Design review of the part built by this model. Coordinates are the model's own, in mm. A direction names the side the tool comes from. Coordinates: 2 decimals unless noted, no trailing zeros. Loops run counter-clockwise (first coordinate to the right, second up) from the corner with the lowest first, then second, coordinate; pieces in that order, holes last. Notation, with made-up numbers: M 14,-25 L 19,-25 A34 cw 19,10 Z; hole C 48,78.5 d10. An arc over 180 degrees is marked long. Put each result on its own line as item: value. Start each with the question number.
(1) The part is to be moulded in two halves that separate along Z. For faces 5 (the flat face through (8.71, -17.16, -3.14)), 6 (the cylindrical face through (13.768, 14.235, -2.872)), say which applies: +Z half, -Z half, draft (parallel to the pull), parting line (faces both ways), or undercut.
(2) For probe 1 along Z at (x, y) = (7.7, -12.5); probe 2 along Y at (x, z) = (14.25, -3.1); probe 3 along Y at (x, z) = (4.25, -3.25), list the stretches that pass through material, from the lowest coordinate up. Write a range as [from, to].
(3) Take a section at A-A, the plane z = -7. Give the boundary of the cut face in (x, y).
(4) Take a section at D-D, the plane x = 13.5. Give the boundary of the cut face in (y, z).
(5) Take a section at B-B, the plane x = 9. Give the boundary of the cut face in (y, z), then the cut area to 3 significant figures.
(6) Clearance check with a flat-ended pin moving along its axis: pin 1 (0.5 mm diameter, centred on y = 12.5, z = -4, fed in from +X). State where the tip first meets the part, or that it passes through.
(7) Take a section at C-C, the plane y = -6. Give the boundary of the cut face in (x, z).
(8) For faces 1 (the flat face through (8.71, 17.16, -3.14)), 2 (the flat face through (10.8, 24, -3)), 3 (the flat face through (10.8, -24, -3)), 4 (the flat face through (9.8, 12, -5)), list the 3-axis set-ups (+Z, -Z, +X, -X, +Y, -Y) from which the entire face can be reached by the end or side of a thin tool; tool diameter is ignored.
```python
from build123d import *

# Parameters (mm, degrees)
ESQUISSE1_W                           = 15
ESQUISSE1_H                           = 10
BOSS_EXTRU_1_DEPTH                    = 25
ENL_VEMENT_START                      = -6.2
ENL_VEMENT_DE_MATI_RE_BALAYAGE1_DEPTH = 6.2
ENL_V_MAT_EXTRU_1_REACH               = 32.822
ESQUISSE4_R                           = 1.75
ENL_V_MAT_EXTRU_2_REACH               = 32.822
ESQUISSE5_W                           = 2.7
ESQUISSE5_H                           = 5.9


# Read off the part's stored shape, not the designer's step: Enlèvement de matière-Balayage1
with BuildPart() as part:
    # Esquisse1 → Boss.-Extru.1 (new body)
    with BuildSketch(Plane(origin=(0, 0, 0), x_dir=(1, 0, 0), z_dir=(0, 1, 0))):
        with Locations((7.5, 5)):
            Rectangle(ESQUISSE1_W, ESQUISSE1_H)
    extrude(amount=BOSS_EXTRU_1_DEPTH)

    # Enlèvement de matière-Balayage1 outline → Enlèvement de matière-Balayage1 (cut)
    with BuildSketch(Plane.XY.offset(ENL_VEMENT_START)):
        with BuildLine():
            Line((10.8, 25), (10.8, 22.058471581))
            ThreePointArc((10.8, 22.058471581), (10.4896694, 20.777243155), (9.627466942, 19.780017862))
            Line((9.627466942, 19.780017862), (5.977561393, 17.172942469))
            ThreePointArc((5.977561393, 17.172942469), (4.376328258, 15.320952639), (3.8, 12.941528419))
            Line((3.8, 12.941528419), (3.8, 12.264761516))
            ThreePointArc((3.8, 12.264761516), (4.474960485, 9.702727678), (6.324622072, 7.805798302))
            Line((6.324622072, 7.805798302), (15, 2.600571545))
            Line((15, 2.600571545), (15, 4.466476152))
            Line((15, 4.466476152), (7.14781528, 9.177786983))
            ThreePointArc((7.14781528, 9.177786983), (5.867280336, 10.491045782), (5.4, 12.264761516))
            Line((5.4, 12.264761516), (5.4, 12.941528419))
            ThreePointArc((5.4, 12.941528419), (5.798996486, 14.58882211), (6.907542503, 15.870968915))
            Line((6.907542503, 15.870968915), (10.557448052, 18.478044308))
            ThreePointArc((10.557448052, 18.478044308), (11.912337628, 20.045112625), (12.4, 22.058471581))
            Line((12.4, 22.058471581), (12.4, 25))
            Line((12.4, 25), (10.8, 25))
        make_face()
    extrude(amount=ENL_VEMENT_DE_MATI_RE_BALAYAGE1_DEPTH, mode=Mode.SUBTRACT)

    # Esquisse4 → Enlèv. mat.-Extru.1 (cut, up to next)
    with BuildSketch(Plane(origin=(15, 0, 0), x_dir=(0, 0, -1), z_dir=(1, 0, 0)), mode=Mode.PRIVATE) as enl_v_mat_extru_1_sk1:
        with Locations((3.1, 12.5)):
            Circle(ESQUISSE4_R)
    enl_v_mat_extru_1_tool1 = extrude(enl_v_mat_extru_1_sk1.sketch, amount=-ENL_V_MAT_EXTRU_1_REACH, mode=Mode.PRIVATE) & part.part
    add(enl_v_mat_extru_1_tool1.solids().sort_by_distance((15, 12.5, -3.1))[0], mode=Mode.SUBTRACT)

    # Esquisse5 → Enlèv. mat.-Extru.2 (cut, up to next)
    with BuildSketch(Plane.XY, mode=Mode.PRIVATE) as enl_v_mat_extru_2_sk1:
        with Locations((11.15, 12.5)):
            Rectangle(ESQUISSE5_W, ESQUISSE5_H)
    enl_v_mat_extru_2_tool1 = extrude(enl_v_mat_extru_2_sk1.sketch, amount=-ENL_V_MAT_EXTRU_2_REACH, mode=Mode.PRIVATE) & part.part
    add(enl_v_mat_extru_2_tool1.solids().sort_by_distance((11.15, 12.5, 0))[0], mode=Mode.SUBTRACT)

    # Symétrie1: part across plane


with BuildPart() as part_1:
    add(part.part)
    add(part.part.mirror(Plane(origin=(0, 0, 0), x_dir=(0, 0, 1), z_dir=(0, -1, 0))))


solid = part_1.part
```
Computed values:
1. face 5: draft
1. face 6: undercut
2. probe 1: z = [-10, -4.85], [-1.35, 0]
2. probe 2: y = [-25, -14.25], [-10.75, -4.92], [-3.05, 3.05], [4.92, 10.75], [14.25, 25]
2. probe 3: y = [-25, -15.06], [-10.15, 10.15], [15.06, 25]
3. outline: M 0,-25 L 15,-25 L 15,25 L 0,25 Z; hole M 9.8,-15.45 L 12.5,-15.45 L 12.5,-9.55 L 9.8,-9.55 Z; hole M 9.8,9.55 L 12.5,9.55 L 12.5,15.45 L 9.8,15.45 Z
4. outline: M -25,-10 L 25,-10 L 25,0 L 5.37,0 L 5.37,-6.2 L 3.5,-6.2 L 3.5,0 L -3.5,0 L -3.5,-6.2 L -5.37,-6.2 L -5.37,0 L -25,0 Z; hole C -12.5,-3.1 d3.5; hole C 12.5,-3.1 d3.5
5. outline: M -25,-10 L 25,-10 L 25,0 L 19.33,0 L 19.33,-6.2 L 17.37,-6.2 L 17.37,0 L 8.07,0 L 8.07,-6.2 L 6.2,-6.2 L 6.2,0 L -6.2,0 L -6.2,-6.2 L -8.07,-6.2 L -8.07,0 L -17.37,0 L -17.37,-6.2 L -19.33,-6.2 L -19.33,0 L -25,0 Z; hole C -12.5,-3.1 d3.5; hole C 12.5,-3.1 d3.5
5. area: 433 mm^2
6. pin 1: stops at x = 3.8
7. outline: M 0,-10 L 15,-10 L 15,0 L 12.44,0 L 12.44,-6.2 L 9.33,-6.2 L 9.33,0 L 0,0 Z
8. face 1: +Z
8. face 2: +Z, +Y
8. face 3: +Z, -Y
8. face 4: +Z, -Z
